Can you work these out from the model? Positions are in its coordinate system, mm. Face numbers are marked on the shaded views. A direction names the side the tool comes from. Coordinates: 2 decimals unless noted, no trailing zeros. Loops run counter-clockwise (first coordinate to the right, second up) from the corner with the lowest first, then second, coordinate; pieces in that order, holes last. Notation, with made-up numbers: (57.5, -31.5) -> (105.5, -31.5) arc R25 cw to (105.5, -18.5) -> close; hole circle Ø9 at (54.5, -34). An arc over 180 degrees is marked (long way). Use one line per item in the form item = value. Start each with the question number.
(1) On a 3-axis mill with a long thin cutter (end or side, diameter ignored), from which of +Z, -Z, +X, -X, +Y, -Y can I reach the whole of each face in a straight line? I mean the marked faces 4, 5 and 6. Say none if no direction works.
(2) Imagine slicing it at C-C (z = 7). List the corners of the cut face in (x, y) for me.
(3) Imagine slicing it at B-B (x = -17). List the corners of the cut face in (y, z) for me, plus the area to 3 significant figures.
(4) Thinking about a two-plate mould opening in Z: for the marked faces 1, 2 and 3, which applies, released by +Z, released by -Z, zero draft, split by the parting line, or undercut?
(5) Imagine slicing it at D-D (x = 9.5). List the corners of the cut face in (y, z) for me.
(6) I'm going to push a flat-ended pin straight in: pin 1 (6.5 mm diameter, centred on x = 17, y = 1.5, fed in from +Z). Where does the tip first touch, or does it pass through?
(7) I need wall thicknesses on line 1 (X direction, y = 0, z = 4.2); line 2 (X direction, y = 0.5, z = 8.75); line 3 (Y direction, x = 18, z = 3.05). Which ranges of each line are inside material? Lowest first, please. Write a range as [from, to].
(8) Imagine slicing it at A-A (y = 0). List the corners of the cut face in (x, z) for me.
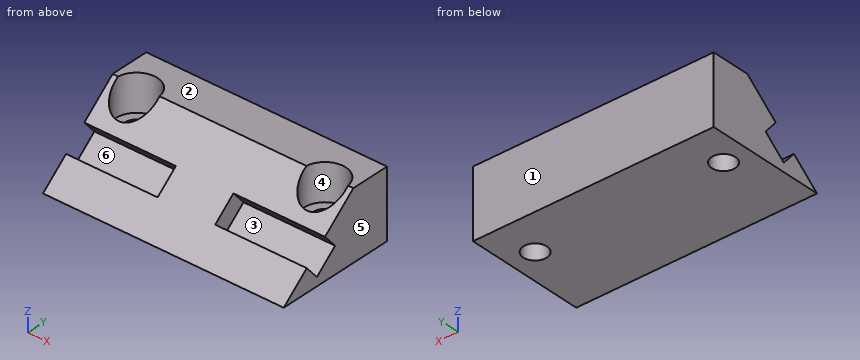
```python
from build123d import *

# Parameters (mm, degrees)
EX_BODY_DEPTH       = 46
SK_SKINBOLTS_R      = 2.25
CUT_SKINBOLTS_DEPTH = 13
SK_BOLTHEADS_R      = 4
CUT_BOLTHEADS_DEPTH = 7
CUT_PLUGL_DEPTH     = 17.5
CUT_PLUGR_DEPTH     = 17.5


with BuildPart() as part:
    # SK_Body → EX_Body (new body)
    with BuildSketch(Plane(origin=(-23, 0, 0), x_dir=(0, 0, -1), z_dir=(1, 0, 0))):
        Polygon((0, -14.989146791), (-13, 0.503649913), (-13, 8), (0, 8), align=None)
    extrude(amount=EX_BODY_DEPTH)

    # SK_SkinBolts → CUT_SkinBolts (cut)
    with BuildSketch(Plane.XY):
        with Locations(Location((18, 0, 0), (0, 0, 167.065065628))):
            Circle(SK_SKINBOLTS_R)
        with Locations(Location((-18, 0, 0), (0, 0, 167.065065628))):
            Circle(SK_SKINBOLTS_R)
    extrude(amount=CUT_SKINBOLTS_DEPTH, mode=Mode.SUBTRACT)

    # SK_BoltHeads → CUT_BoltHeads (cut)
    with BuildSketch(Plane.XY.offset(6)):
        with Locations(Location((18, 0, 0), (0, 0, 172.766546712))):
            Circle(SK_BOLTHEADS_R)
        with Locations(Location((-18, 0, 0), (0, 0, 172.766546712))):
            Circle(SK_BOLTHEADS_R)
    extrude(amount=CUT_BOLTHEADS_DEPTH, mode=Mode.SUBTRACT)

    # SK_PlugL → CUT_PlugL (cut)
    with BuildSketch(Plane(origin=(5.5, 0, 0), x_dir=(0, 0, -1), z_dir=(1, 0, 0))):
        Polygon((-4.304897282, -9.858769989), (-7.711671614, -5.798734441), (-5.030516063, -3.548977807), (-1.623741731, -7.609013355), align=None)
    extrude(amount=CUT_PLUGL_DEPTH, mode=Mode.SUBTRACT)

    # SK_PlugR → CUT_PlugR (cut)
    with BuildSketch(Plane(origin=(-5.5, 0, 0), x_dir=(0, 0, -1), z_dir=(1, 0, 0))):
        Polygon((-4.304897282, -9.858769989), (-7.711671614, -5.798734441), (-5.030516063, -3.548977807), (-1.623741731, -7.609013355), align=None)
    extrude(amount=-CUT_PLUGR_DEPTH, mode=Mode.SUBTRACT)


solid = part.part
```
Worked out:
q1.face_4 = +Z
q1.face_5 = +Z, -Z, +X, +Y, -Y
q1.face_6 = -X
q2.outline = (-23, -5.2) -> (-5.5, -5.2) -> (-5.5, -6.65) -> (5.5, -6.65) -> (5.5, -5.2) -> (23, -5.2) -> (23, 8) -> (-23, 8) -> close; hole circle Ø8 at (-18, 0); hole circle Ø8 at (18, 0)
q3.outline = (-14.99, 0) -> (-2.02, 0) -> (-2.02, 6) -> (-3.87, 6) -> (-3.87, 9.33) -> (-5.8, 7.71) -> (-3.55, 5.03) -> (-7.61, 1.62) -> (-9.86, 4.3) -> close; (2.02, 0) -> (8, 0) -> (8, 13) -> (3.87, 13) -> (3.87, 6) -> (2.02, 6) -> close
q3.area = 109 mm2
q4.face_1 = zero draft
q4.face_2 = released by +Z
q4.face_3 = undercut
q5.outline = (-14.99, 0) -> (8, 0) -> (8, 13) -> (0.5, 13) -> (-5.8, 7.71) -> (-3.55, 5.03) -> (-7.61, 1.62) -> (-9.86, 4.3) -> close
q6.pin_1 = 13
q7.line_1 = [-23, -20.25], [-15.75, 15.75], [20.25, 23]
q7.line_2 = [-23, -21.97], [-14.03, 14.03], [21.97, 23]
q7.line_3 = [-11.35, -8.81], [-5.91, -2.25], [2.25, 8]
q8.outline = (-23, 0) -> (-20.25, 0) -> (-20.25, 6) -> (-22, 6) -> (-22, 12.58) -> (-23, 12.58) -> close; (-15.75, 0) -> (15.75, 0) -> (15.75, 6) -> (14, 6) -> (14, 12.58) -> (-14, 12.58) -> (-14, 6) -> (-15.75, 6) -> close; (20.25, 0) -> (23, 0) -> (23, 12.58) -> (22, 12.58) -> (22, 6) -> (20.25, 6) -> close
